The model under review builds one solid part; all positions refer to its coordinate system, in mm. A direction names the side the tool comes from. Round coordinates to 2 decimals unless told otherwise and drop trailing zeros. Loops run counter-clockwise (first coordinate to the right, second up) from the corner with the lowest first, then second, coordinate; pieces in that order, holes last. Notation, with made-up numbers: (26.5, 47) -> (43.5, 47) arc R22 ccw to (43.5, 67) -> close; hole circle Ø4 at (32.25, -3). An arc over 180 degrees is marked (long way). Return JSON: item names as keys, results as strings. Group by question number.
```python
from build123d import *
from build123d.topology import SkipClean

# Parameters (mm, degrees)
SKETCH1_R           = 6.45
BOSS_EXTRUDE1_DEPTH = 15
SKETCH2_W           = 5
SKETCH2_H           = 3
CUT_EXTRUDE3_DEPTH  = 5
SKETCH4_R           = 1.5
CUT_EXTRUDE4_DEPTH  = 56.180796325
SKETCH5_R           = 3
CUT_EXTRUDE5_DEPTH  = 4
CUT_EXTRUDE6_START  = -80
CUT_EXTRUDE6_DEPTH  = 80


with BuildPart() as part:
    # Sketch1 → Boss-Extrude1 (new body)
    with BuildSketch(Plane.XY):
        with BuildLine():
            Line((0, 23), (0, 37))
            Line((0, 37), (12.859510911, 37))
            Line((12.859510911, 37), (12.859510911, 27))
            ThreePointArc((12.859510911, 27), (20.383390121, 21.88342816), (26.020458433, 14.741192754))
            Line((26.020458433, 14.741192754), (28.050458433, 14.741192754))
            Line((28.050458433, 14.741192754), (28.050458433, 9.460443964))
            ThreePointArc((28.050458433, 9.460443964), (34.500458433, 11.45), (40.950458433, 9.460443964))
            Line((40.950458433, 9.460443964), (40.950458433, 35))
            Line((40.950458433, 35), (50.950458433, 35))
            Line((50.950458433, 35), (50.950458433, -35))
            Line((50.950458433, -35), (40.950458433, -35))
            Line((40.950458433, -35), (40.950458433, -9.460443964))
            ThreePointArc((40.950458433, -9.460443964), (34.500458433, -11.45), (28.050458433, -9.460443964))
            Line((28.050458433, -9.460443964), (28.050458433, -14.741192754))
            Line((28.050458433, -14.741192754), (26.020458433, -14.741192754))
            ThreePointArc((26.020458433, -14.741192754), (20.383390121, -21.88342816), (12.859510911, -27))
            Line((12.859510911, -27), (12.859510911, -37))
            Line((12.859510911, -37), (0, -37))
            Line((0, -37), (0, -23))
            ThreePointArc((0, -23), (23, 0), (0, 23))
        make_face()
        with Locations(Location((34.500458433, 0, 0), (0, 0, 180))):
            Circle(SKETCH1_R, mode=Mode.SUBTRACT)
    boss_extrude1 = extrude(amount=BOSS_EXTRUDE1_DEPTH)

    # Sketch2 → Cut-Revolve1 (revolve, cut)
    with BuildSketch(Plane.ZY):
        with Locations((7.5, 24.5)):
            Rectangle(SKETCH2_W, SKETCH2_H)
    cut_revolve1 = revolve(axis=Axis((0, 0, 15), (0, 0, -1)), mode=Mode.SUBTRACT)

    # Sketch3 → Cut-Extrude3 (cut)
    with BuildSketch(Plane(origin=(50.950458433, 0, 0), x_dir=(0, 0, -1), z_dir=(1, 0, 0))):
        with BuildLine():
            Line((-12.5, -25), (-12.5, 25))
            ThreePointArc((-12.5, 25), (-7.5, 30), (-2.5, 25))
            Line((-2.5, 25), (-2.5, -25))
            ThreePointArc((-2.5, -25), (-7.5, -30), (-12.5, -25))
        make_face()
    extrude(amount=-CUT_EXTRUDE3_DEPTH, mode=Mode.SUBTRACT)

    # Sketch4 → Cut-Extrude4 (cut, symmetric)
    with BuildSketch(Plane(origin=(12.859510911, 0, 0), x_dir=(0, 0, -1), z_dir=(1, 0, 0))):
        with Locations((-7.333431897, 32)):
            Circle(SKETCH4_R)
        with Locations((-7.333431897, -32)):
            Circle(SKETCH4_R)
    cut_extrude4 = extrude(amount=CUT_EXTRUDE4_DEPTH, both=True, mode=Mode.SUBTRACT)

    # Sketch5 → Cut-Extrude5 (cut)
    with BuildSketch(Plane(origin=(12.859510911, 0, 0), x_dir=(0, 0, -1), z_dir=(1, 0, 0))):
        with Locations((-7.5, 32)):
            Circle(SKETCH5_R)
        with Locations(Location((-7.5, -32, 0), (0, 0, 180))):
            Circle(SKETCH5_R)
    cut_extrude5 = extrude(amount=-CUT_EXTRUDE5_DEPTH, mode=Mode.SUBTRACT)

    # Mirror1: Boss-Extrude1, Cut-Revolve1, Cut-Extrude4, Cut-Extrude5 across plane
    add(boss_extrude1.mirror(Plane.ZY))
    add(cut_revolve1.mirror(Plane.ZY), mode=Mode.SUBTRACT)
    add(cut_extrude4.mirror(Plane.ZY), mode=Mode.SUBTRACT)
    add(cut_extrude5.mirror(Plane.ZY), mode=Mode.SUBTRACT)

    # Sketch6 → Cut-Extrude6 (cut)
    with SkipClean():  # the faces are left unmerged after this step: merging them gives an invalid solid
        with BuildSketch(Plane.XY.offset(15).offset(CUT_EXTRUDE6_START)):
            with BuildLine():
                Line((-40.950458433, 9.460443964), (-40.950458433, 38.741811421))
                Line((-40.950458433, 38.741811421), (-62.772471418, 38.741811421))
                Line((-62.772471418, 38.741811421), (-62.772471418, -39.471412389))
                Line((-62.772471418, -39.471412389), (-40.950458433, -39.471412389))
                Line((-40.950458433, -39.471412389), (-40.950458433, -9.460443964))
                ThreePointArc((-40.950458433, -9.460443964), (-45.950458433, 0), (-40.950458433, 9.460443964))
            make_face()
        extrude(amount=CUT_EXTRUDE6_DEPTH, mode=Mode.SUBTRACT)


solid = part.part
```
1. Draft analysis for pull direction Y (two halves, no side actions). For faces 1 (the face through (48, 0, 2.5)), 2 (the face through (48.5, 30, 7.6)), 3 (the face through (-12.86, -35.3, 7.4)), 4 (the face through (46, 35, 7)), state which applies: pulls with the +Y half, pulls with the -Y half, needs draft (parallel to the pull), parting line crosses it, or undercut.
2. We need section B-B, the plane x = -4. Write out the cut boundary in (y, z).
3. We need section D-D, the plane y = 18. Write out the cut boundary in (x, z), then the cut area to 3 significant figures.
4. Tool access review of faces 5 (the face through (-28.05, -12, 7)), 6 (the face through (20.29, 21.97, 7.4)), 7 (the face through (-27, 14.741, 7)): name each direction out of +Z, -Z, +X, -X, +Y, -Y from which nothing blocks a thin tool from reaching the whole face with its end or side.
5. Wall thickness on line 1 (Z direction, x = 47, y = 32); line 2 (X direction, y = -29, z = 6.5); line 3 (Y direction, x = 0, z = 1.4): over which ranges is each line inside the solid? List them lowest first.
6. We need section C-C, the plane x = -35.5. Write out the cut boundary in (y, z), then the cut area to 3 significant figures.
7. For P1, Ø8, axis at x = -19, z = 10, coming from the -Y side; P2, Ø3, axis at y = 34.5, z = 6.5, coming from the -X side; P3, Ø5, axis at y = 5, z = 4.5, coming from the -X side, all flat-tipped, find the tip position at first contact; note any pin that passes through.
8. We need section A-A, the plane y = 0. Write out the cut boundary in (x, z).
Check sheet entries:
{
 "1": {"face 1": "undercut", "face 2": "undercut", "face 3": "needs draft", "face 4": "pulls with the +Y half"},
 "2": {"outline": "(-37, 0) -> (-22.65, 0) -> (-22.65, 5) -> (-25.69, 5) -> (-25.69, 10) -> (-22.65, 10) -> (-22.65, 15) -> (-37, 15) -> close; (22.65, 0) -> (37, 0) -> (37, 15) -> (22.65, 15) -> (22.65, 10) -> (25.69, 10) -> (25.69, 5) -> (22.65, 5) -> close; hole circle Ø3 at (-32, 7.33); hole circle Ø3 at (32, 7.33)"},
 "3": {"outline": "(-23.88, 0) -> (-14.32, 0) -> (-14.32, 5) -> (-18.76, 5) -> (-18.76, 10) -> (-14.32, 10) -> (-14.32, 15) -> (-23.88, 15) -> close; (14.32, 0) -> (23.88, 0) -> (23.88, 15) -> (14.32, 15) -> (14.32, 10) -> (18.76, 10) -> (18.76, 5) -> (14.32, 5) -> close; (40.95, 0) -> (50.95, 0) -> (50.95, 2.5) -> (45.95, 2.5) -> (45.95, 12.5) -> (50.95, 12.5) -> (50.95, 15) -> (40.95, 15) -> close", "area": "342 mm²"},
 "4": {"face 5": "+Z, -Z, -Y", "face 6": "+Z, -Z, +Y", "face 7": "+Z, -Z, -X, +Y"},
 "5": {"line 1": "z = 0 to 5.83, 8.83 to 15", "line 2": "x = -12.86 to 12.86, 40.95 to 45.95", "line 3": "y = -37 to -23, 23 to 37"},
 "6": {"outline": "(-11.41, 0) -> (-6.37, 0) -> (-6.37, 15) -> (-11.41, 15) -> close; (6.37, 0) -> (11.41, 0) -> (11.41, 15) -> (6.37, 15) -> close", "area": "151 mm²"},
 "7": {"P1": "stops at y = -25.87", "P2": "stops at x = -12.86", "P3": "stops at x = -45.67"},
 "8": {"outline": "(-45.95, 0) -> (-40.95, 0) -> (-40.95, 15) -> (-45.95, 15) -> close; (-28.05, 0) -> (-23, 0) -> (-23, 5) -> (-26, 5) -> (-26, 10) -> (-23, 10) -> (-23, 15) -> (-28.05, 15) -> close; (23, 0) -> (28.05, 0) -> (28.05, 15) -> (23, 15) -> (23, 10) -> (26, 10) -> (26, 5) -> (23, 5) -> close; (40.95, 0) -> (50.95, 0) -> (50.95, 2.5) -> (45.95, 2.5) -> (45.95, 12.5) -> (50.95, 12.5) -> (50.95, 15) -> (40.95, 15) -> close"}
}
